CAD build for the part. Positions are in the model's coordinates, mm. Give positions to 0.01 mm unless a question says otherwise; leave off trailing zeros. Loops run counter-clockwise (first coordinate to the right, second up) from the corner with the lowest first, then second, coordinate; pieces in that order, holes last.
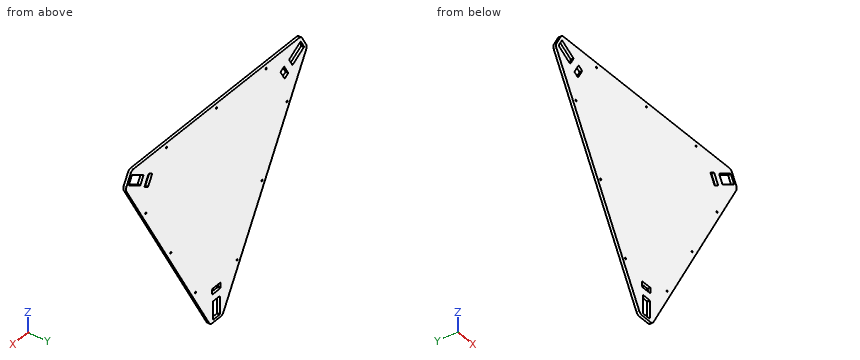
```python
from build123d import *

# Parameters (mm, degrees)
SKETCH_1_W         = 20.5
SKETCH_1_H         = 40.5
SKETCH_1_W_2       = 25
SKETCH_1_H_2       = 12.5
EXTRUDE_1388_DEPTH = 3
FILLET_1_R         = 10
FILLET_2_R         = 1.5
HOLE_WIZARD_3_5_D  = 3.5


with BuildPart() as part:
    # Эскиз1 → Extrude 1388 (new, symmetric)
    with BuildSketch(Plane(origin=(0, 0, 0), x_dir=(1, 0, 0), z_dir=(0, 1, 0))):
        Polygon((273.664027596, -136.63804004), (18.5, 305.31902002), (-18.5, 305.31902002), (-273.664027596, -136.63804004), (-255.164027596, -168.68097998), (255.164027596, -168.68097998), align=None)
        Polygon((219.01884632, -138.286270399), (254.092875173, -158.536270399), (264.342875173, -140.782749621), (229.26884632, -120.532749621), align=None, mode=Mode.SUBTRACT)
        with Locations((0, 279.06902002)):
            Rectangle(SKETCH_1_W, SKETCH_1_H, mode=Mode.SUBTRACT)
        Polygon((-229.26884632, -120.532749621), (-264.342875173, -140.782749621), (-254.092875173, -158.536270399), (-219.01884632, -138.286270399), align=None, mode=Mode.SUBTRACT)
        Polygon((216.537439859, -110.584192463), (204.037439859, -132.234827557), (193.212122312, -125.984827557), (205.712122312, -104.334192463), align=None, mode=Mode.SUBTRACT)
        with Locations((0, 236.56902002)):
            Rectangle(SKETCH_1_W_2, SKETCH_1_H_2, mode=Mode.SUBTRACT)
        Polygon((-204.037439859, -132.234827557), (-216.537439859, -110.584192463), (-205.712122312, -104.334192463), (-193.212122312, -125.984827557), align=None, mode=Mode.SUBTRACT)
    extrude(amount=EXTRUDE_1388_DEPTH, both=True)

    # Скругление1
    fillet_1_edges = [part.edges().sort_by_distance(p)[0] for p in [
        (255.164027596, 0, 168.68097998),
        (-255.164027596, 0, 168.68097998),
        (-273.664027596, 0, 136.63804004),
        (-18.5, 0, -305.31902002),
        (18.5, 0, -305.31902002),
        (273.664027596, 0, 136.63804004),
    ]]
    fillet(fillet_1_edges, radius=FILLET_1_R)

    # Скругление2
    fillet_2_edges = [part.edges().sort_by_distance(p)[0] for p in [
        (10.25, 0, -258.81902002),
        (10.25, 0, -299.31902002),
        (-10.25, 0, -299.31902002),
        (-10.25, 0, -258.81902002),
        (12.5, 0, -230.31902002),
        (12.5, 0, -242.81902002),
        (-12.5, 0, -242.81902002),
        (-12.5, 0, -230.31902002),
        (229.26884632, 0, 120.532749621),
        (219.01884632, 0, 138.286270399),
        (254.092875173, 0, 158.536270399),
        (264.342875173, 0, 140.782749621),
        (-219.01884632, 0, 138.286270399),
        (-229.26884632, 0, 120.532749621),
        (-264.342875173, 0, 140.782749621),
        (-254.092875173, 0, 158.536270399),
        (193.212122312, 0, 125.984827557),
        (204.037439859, 0, 132.234827557),
        (216.537439859, 0, 110.584192463),
        (205.712122312, 0, 104.334192463),
        (-205.712122312, 0, 104.334192463),
        (-216.537439859, 0, 110.584192463),
        (-204.037439859, 0, 132.234827557),
        (-193.212122312, 0, 125.984827557),
    ]]
    fillet(fillet_2_edges, radius=FILLET_2_R)

    # Отверстия 3,5мм (through all)
    with Locations(Plane(origin=(0, 3, 0), x_dir=(1, 0, 0), z_dir=(0, 1, 0))):
        with Locations((-137.42175976, 79.34048999), (-62.42175976, 209.244300558), (62.42175976, 209.244300558), (137.42175976, 79.34048999), (212.42175976, -50.563320578), (150, -158.68097998), (0, -158.68097998), (-150, -158.68097998), (-212.42175976, -50.563320578)):
            Hole(HOLE_WIZARD_3_5_D / 2)


solid = part.part
```
1. Saw through at A-A, the plane z = -131. List the corners of the cut face in (x, y), and give its area (3 significant figures).
Responses:
outline: (-119.14, -3) - (119.14, -3) - (119.14, 3) - (-119.14, 3) - close
area: 1,430 mm2
2. Drop flat-ended pins along their axis: pin 1 (3 mm diameter, centred on x = -212.42, z = 50.56, fed in from +Y); pin 2 (4.5 mm diameter, centred on x = -62.42, z = -209.24, fed in from -Y); pin 3 (1 mm diameter, centred on x = 77.5, y = 2.5, fed in from -Z); pin 4 (3 mm diameter, centred on y = 1.5, z = -235, fed in from -X). Give the stop position or say it passes through.
Responses:
pin 1: passes through
pin 2: stops at y = -3
pin 3: stops at z = -203.99
pin 4: stops at x = -59.96
3. Saw through at C-C, the plane y = 1.7. Count the separate pieces of the cut face and the enclosed holes in it, and give its area (3 significant figures).
Responses:
separate pieces: 1
enclosed holes: 15
area: 143,000 mm2
4. Probe line 1 along Z through (x, y) = (-6, -0.75); line 2 along Z through (x, y) = (-150, 1.55); line 3 along X through (y, z) = (1.8, 110.5). List the from-to ranges inside material, lowest first.
Responses:
line 1: z = -305.32 to -299.32, -258.82 to -242.82, -230.32 to 168.68
line 2: z = -77.55 to 156.93, 160.43 to 168.68
line 3: x = -258.57 to -215.85, -202.15 to 202.15, 215.85 to 258.57
5. Saw through at B-B, the plane x = 165.5. List the corners of the cut face in (y, z), and give its area (3 significant figures).
Responses:
outline: (-3, -50.71) - (3, -50.71) - (3, 168.68) - (-3, 168.68) - close
area: 1,320 mm2
